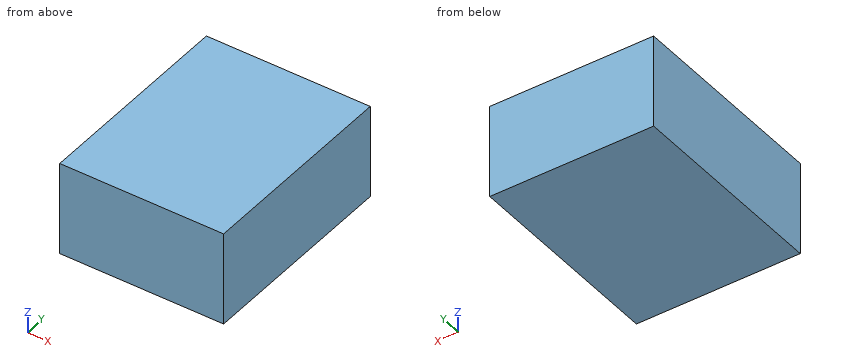
```python
from build123d import *

# Parameters (mm, degrees)
F0_W     = 440
F0_H     = 250
F0_W_2   = 434
F0_H_2   = 244
F1_DEPTH = 277
F2_W     = 440
F2_H     = 250
F3_DEPTH = 3
F4_W     = 440
F4_H     = 250
F5_DEPTH = 3


with BuildPart() as f1:
    # F0 (on Front) → F1 (new body, symmetric)
    with BuildSketch(Plane.XZ):
        with Locations((0, 125)):
            Rectangle(F0_W, F0_H)
        with Locations((0, 125)):
            Rectangle(F0_W_2, F0_H_2, mode=Mode.SUBTRACT)
    extrude(amount=F1_DEPTH, both=True)

    # F2 (on face) → F3 (join)
    with BuildSketch(Plane.XZ.offset(277)):
        with Locations((0, 125)):
            Rectangle(F2_W, F2_H)
    extrude(amount=F3_DEPTH)

    # F4 (on face) → F5 (join)
    with BuildSketch(Plane(origin=(0, 277, 0), x_dir=(-1, 0, 0), z_dir=(0, 1, 0))):
        with Locations((0, 125)):
            Rectangle(F4_W, F4_H)
    extrude(amount=F5_DEPTH)


solid = f1.part
```
For this review, take the finished solid that the model builds, in its own axes (mm). Give positions to 0.01 mm unless a question says otherwise; leave off trailing zeros. Order: outer loops, then holes, each group sorted by start corner. A loop starts at its lowest first (then second) coordinate and runs counter-clockwise, first axis right, second up.
1) Take a section at A-A (x = -71). Give the boundary of the cut face in (y, z), then the cut area to 3 significant figures.
2) Take a section at B-B (y = -221.5). Give the boundary of the cut face in (x, z).
3) Wall thickness on line 1 (X direction, y = -168.5, z = 33.5); line 2 (Z direction, x = -173.5, y = 245); line 3 (Y direction, x = -51.5, z = 113.5): over which ranges is each line inside the solid? List them lowest first.
Derived:
1. outline: (-280, 0) - (280, 0) - (280, 250) - (-280, 250) - close; hole (-277, 3) - (277, 3) - (277, 247) - (-277, 247) - close
1. area: 4,820 mm2
2. outline: (-220, 0) - (220, 0) - (220, 250) - (-220, 250) - close; hole (-217, 3) - (217, 3) - (217, 247) - (-217, 247) - close
3. line 1: x = -220 to -217, 217 to 220
3. line 2: z = 0 to 3, 247 to 250
3. line 3: y = -280 to -277, 277 to 280
